from build123d import *

# Parameters (mm, degrees)
SKETCH021_R            = 1.6
PAD005_DEPTH           = 4
FILLET_R               = 5
SKETCH022_W            = 3
SKETCH022_H            = 80
POCKET010_DEPTH        = 4.001
LINEARPATTERN002_COUNT = 7
LINEARPATTERN002_PITCH = 16.666667


with BuildPart() as part:
    # Sketch021 (on Face1 of ShapeBinder002) → Pad005 (new body)
    with BuildSketch(Plane.XY.offset(41.135521)):
        Polygon((189, 120.6), (189, 2), (201, 2), (201, -4), (207, -4), (207, 2), (307, 2), (307, -4), (313, -4), (313, 2), (325, 2), (325, 120.6), align=None)
        with Locations((204, -1)):
            Circle(SKETCH021_R, mode=Mode.SUBTRACT)
        with Locations((310, -1)):
            Circle(SKETCH021_R, mode=Mode.SUBTRACT)
        with Locations((204, 116.85)):
            Circle(SKETCH021_R, mode=Mode.SUBTRACT)
        with Locations((310, 116.85)):
            Circle(SKETCH021_R, mode=Mode.SUBTRACT)
    extrude(amount=PAD005_DEPTH)

    # Fillet
    fillet_edges = [part.edges().sort_by_distance(p)[0] for p in [
        (207, 2, 43.135521),
        (201, 2, 43.135521),
        (307, 2, 43.135521),
        (313, 2, 43.135521),
    ]]
    fillet(fillet_edges, radius=FILLET_R)

    # Sketch022 (on Face5 of Fillet) → Pocket010 (cut, through all)
    with BuildSketch(Plane.XY.offset(45.135521)):
        with Locations((203.968842, 61.629364)):
            Rectangle(SKETCH022_W, SKETCH022_H)
    pocket010 = extrude(amount=-POCKET010_DEPTH, mode=Mode.SUBTRACT)

    # LinearPattern002: Pocket010 ×7
    with Locations(*[(i * LINEARPATTERN002_PITCH, 0, 0) for i in range(1, LINEARPATTERN002_COUNT)]):
        add(pocket010, mode=Mode.SUBTRACT)


solid = part.part
Design review of the part built by this model. Coordinates are the model's own, in mm. A direction names the side the tool comes from. Round coordinates to 2 decimals unless told otherwise and drop trailing zeros. Loops run counter-clockwise (first coordinate to the right, second up) from the corner with the lowest first, then second, coordinate; pieces in that order, holes last. Notation, with made-up numbers: (29.25, 7.5) - (47.25, 7.5) arc R29 cw to (47.25, 30.5) - close; hole circle Ø10 at (35, 89). An arc over 180 degrees is marked (long way). One line per item, written item: value. Start each with the question number.
1) Draft analysis for pull direction Y (two halves, no side actions). For faces 4 (the flat face through (325, 60, 43)), 5 (the flat face through (221, 21.629, 43)), 6 (the cylindrical face through (315, 1, 43)), state which applies: +Y half, -Y half, draft (parallel to the pull), parting line (faces both ways), or undercut.
2) Insertion check: pin 1 Ø1.5 at (x, z) = (270.5, 44) entering from -Y; pin 2 Ø0.8 at (y, z) = (-3.5, 44) entering from +X; pin 3 Ø0.5 at (y, z) = (-3.5, 44) entering from -X. Each pin has a flat end and moves straight along its axis. Give the tip position at first contact, or say it passes through.
3) To check wall thickness, follow L1, parallel to Y at x = 204, z = 42.4; L2, parallel to X at y = 116.85, z = 43.55; L3, parallel to Y at x = 310, z = 43.05. State the ranges of each line that lie inside material, in increasing order. Write a range as from..to.
4) Consider section A-A on y = 81. Give the number of separate pieces and of enclosed holes in the cut face, then the cut area to 3 significant figures.
5) Consider section B-B on x = 310. Give the boundary of the cut face in (y, z).
6) For faces 1 (the flat face through (221, 101.629, 43)), 2 (the flat face through (192, 2, 43)), 3 (the cylindrical face through (208, 0, 43)), list the 3-axis set-ups (+Z, -Z, +X, -X, +Y, -Y) from which the entire face can be reached by the end or side of a thin tool; tool diameter is ignored.
7) Consider section C-C on y = 116.85. Give the boundary of the cut face in (x, z).
8) Consider section D-D on y = -1. Give the boundary of the cut face in (x, z).
Reported:
1. face 4: draft
1. face 5: undercut
1. face 6: -Y half
2. pin 1: stops at y = 2
2. pin 2: stops at x = 313
2. pin 3: stops at x = 201
3. L1: y = -4..-2.6, 0.6..21.63, 101.63..115.25, 118.45..120.6
3. L2: x = 189..202.4, 205.6..308.4, 311.6..325
3. L3: y = -4..-2.6, 0.6..115.25, 118.45..120.6
4. separate pieces: 8
4. enclosed holes: 0
4. area: 460 mm^2
5. outline: (-4, 41.14) - (-2.6, 41.14) - (-2.6, 45.14) - (-4, 45.14) - close; (0.6, 41.14) - (115.25, 41.14) - (115.25, 45.14) - (0.6, 45.14) - close; (118.45, 41.14) - (120.6, 41.14) - (120.6, 45.14) - (118.45, 45.14) - close
6. face 1: +Z, -Z
6. face 2: +Z, -Z, -X, -Y
6. face 3: +Z, -Z, -Y
7. outline: (189, 41.14) - (202.4, 41.14) - (202.4, 45.14) - (189, 45.14) - close; (205.6, 41.14) - (308.4, 41.14) - (308.4, 45.14) - (205.6, 45.14) - close; (311.6, 41.14) - (325, 41.14) - (325, 45.14) - (311.6, 45.14) - close
8. outline: (200.58, 41.14) - (202.4, 41.14) - (202.4, 45.14) - (200.58, 45.14) - close; (205.6, 41.14) - (207.42, 41.14) - (207.42, 45.14) - (205.6, 45.14) - close; (306.58, 41.14) - (308.4, 41.14) - (308.4, 45.14) - (306.58, 45.14) - close; (311.6, 41.14) - (313.42, 41.14) - (313.42, 45.14) - (311.6, 45.14) - close
